Could you check a few things on this model? Use its own coordinates, in mm. Face numbers are marked on the shaded views. A direction names the side the tool comes from. Give positions to 0.01 mm unless a question says otherwise; leave off trailing zeros. Order: outer loops, then holes, each group sorted by start corner. A loop starts at its lowest first (then second) coordinate and runs counter-clockwise, first axis right, second up. Notation, with made-up numbers: (7.25, 85) - (39.25, 85) arc R19 cw to (39.25, 120) - close; hole circle Ø5 at (25.25, 18). An arc over 180 degrees is marked (long way). One line per question, with ' | ' between items. Start each with the question number.
1. If we mould it in two halves opening along Y, with no side actions, what happens to the marked faces 1, 2 and 3? For each: released by +Y, released by -Y, zero draft, split by the parting line, or undercut.
2. Imagine slicing it at C-C (x = 0). Please give me the cut outline in (y, z), and give its area (3 significant figures).
3. Imagine slicing it at A-A (y = 0). Please give me the cut outline in (x, z).
4. I need wall thicknesses on probe 1 along Y at (x, z) = (-2.25, 14); probe 2 along Y at (x, z) = (0.25, 22); probe 3 along Y at (x, z) = (0.25, 45.5). Which ranges of each line are inside material? Lowest first, please. Write a range as from..to.
5. Which directions (+Z, -Z, +X, -X, +Y, -Y) give clear straight access to the entire face, cutting with the end or side of a thin tool? Please do the marked faces 4, 5 and 6.
6. Imagine slicing it at D-D (y = 13.75). Please give me the cut outline in (x, z), and give its area (3 significant figures).
7. Imagine slicing it at B-B (z = 6). Please give me the cut outline in (x, y), and give its area (3 significant figures).
8. For P1, Ø2, axis at y = 8.5, z = 38, coming from the -X side; P2, Ø3, axis at x = -3, z = 36.5, coming from the -Y side; P3, Ø1.5, axis at x = 3, z = 16, coming from the -Y side; P4, Ø1, axis at y = 1, z = 18, coming from the +X side, each with a flat end and sliding along its axis, tell me the tip position at first contact or that it passes through.
```python
from build123d import *

# Parameters (mm, degrees)
SKETCH_1_R      = 3
EXTRUDE_1_DEPTH = 48
SKETCH_2_R      = 1.75
EXTRUDE_2_DEPTH = 10
EXTRUDE_3_DEPTH = 6.5
CHAMFER_1_SIZE  = 0.5


with BuildPart() as part:
    # 草图1 → 凸台-拉伸1 (new body)
    with BuildSketch(Plane.XY):
        Circle(SKETCH_1_R)
    extrude(amount=EXTRUDE_1_DEPTH)

    # 草图2 → 凸台-拉伸2 (add)
    with BuildSketch(Plane(origin=(0, 0, 0), x_dir=(1, 0, 0), z_dir=(0, 1, 0))):
        with Locations(Location((0, -43, 0), (0, 0, 90))):
            Circle(SKETCH_2_R)
    extrude(amount=EXTRUDE_2_DEPTH)

    # 草图3 → 凸台-拉伸3 (add)
    with BuildSketch(Plane(origin=(0, 10, 0), x_dir=(1, 0, 0), z_dir=(0, 1, 0))):
        Polygon((-1.993644271, -39.820579321), (-3.750281213, -43.136836245), (-1.756636942, -46.316256924), (1.993644271, -46.179420679), (3.750281213, -42.863163755), (1.756636942, -39.683743076), align=None)
    extrude(amount=EXTRUDE_3_DEPTH)

    # 草图4 → 切除-旋转1 (revolve, cut)
    with BuildSketch(Plane(origin=(0, 0, 0), x_dir=(0, 0, -1), z_dir=(1, 0, 0))):
        Polygon((-44.75, 10), (-47.118639965, 11.367534921), (-47.118639965, 10), align=None)
    revolve(axis=Axis((0, 10, 43), (0, -1, 0)), mode=Mode.SUBTRACT)

    # 倒角1
    chamfer_1_edges = [part.edges().sort_by_distance(p)[0] for p in [
        (-3, 0, 0),
        (-3, 0, 48),
    ]]
    chamfer(chamfer_1_edges, length=CHAMFER_1_SIZE)


solid = part.part
```
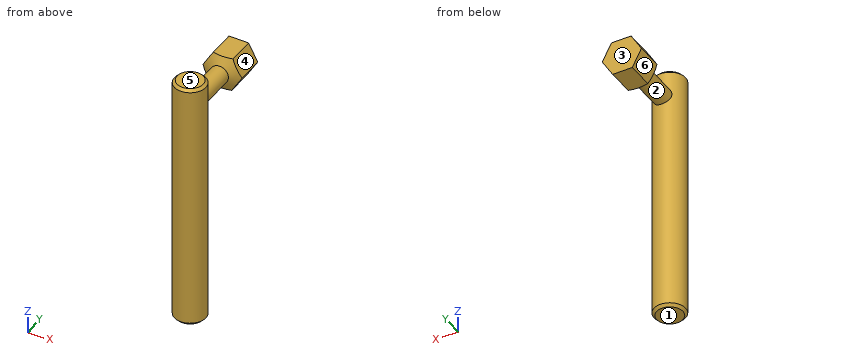
Results found:
1) face 1: zero draft | face 2: undercut | face 3: released by +Y
2) outline: (-3, 0.5) - (-2.5, 0) - (2.5, 0) - (3, 0.5) - (3, 41.25) - (10, 41.25) - (10.87, 39.75) - (16.5, 39.75) - (16.5, 46.25) - (10.87, 46.25) - (10, 44.75) - (3, 44.75) - (3, 47.5) - (2.5, 48) - (-2.5, 48) - (-3, 47.5) - close | area: 353 mm2
3) outline: (-3, 0.5) - (-2.5, 0) - (2.5, 0) - (3, 0.5) - (3, 47.5) - (2.5, 48) - (-2.5, 48) - (-3, 47.5) - close
4) probe 1: y = -1.98..1.98 | probe 2: y = -2.99..2.99 | probe 3: y = -2.99..2.99, 10.44..16.5
5) face 4: +Z, +X, +Y | face 5: +Z, +X, -X, +Y, -Y | face 6: -Z, -X, +Y
6) outline: (-3.75, 43.14) - (-1.99, 39.82) - (1.76, 39.68) - (3.75, 42.86) - (1.99, 46.18) - (-1.76, 46.32) - close | area: 36.6 mm2
7) outline: circle Ø6 at (0, 0) | area: 28.3 mm2
8) P1: passes through | P2: stops at y = -2.6 | P3: stops at y = -1.98 | P4: stops at x = 2.96
